Autodesk Inventor part; units mm, degrees
ref_plane "YZ Plane" through (0, 0, 0) normal (1, 0, 0) x (0, 1, 0)
ref_plane "XZ Plane" through (0, 0, 0) normal (0, 1, 0) x (-1, 0, 0)
ref_plane "XY Plane" through (0, 0, 0) normal (0, 0, 1) x (1, 0, 0)
sketch "Sketch1" plane through (0, 0, 0) normal (0, 1, 0) x (-1, 0, 0)
  line L0 (37.5, 25) -> (-37.5, 25)
  line L1 (-37.5, 25) -> (-37.5, -25)
  line L2 (-37.5, -25) -> (37.5, -25)
  line L3 (37.5, -25) -> (37.5, 25)
  circle A0 centre (-7.5, 7.5) radius 1.75
  circle A1 centre (7.5, -7.5) radius 1.75
  line L4 (-7.5, 7.5) -> (7.5, -7.5) construction
  circle A2 centre (15.5, 15.5) radius 5
  line L5 (15.5, 15.5) -> (-15.5, -15.5) construction
  circle A3 centre (-15.5, -15.5) radius 5
  line L6 (15.5, 15.5) -> (13.8367, 7.6748) construction
  line L7 (30.9543, 4.0364) -> (-3.2809, 11.3133) construction
  circle A4 centre (13.8367, 7.6748) radius 14 construction
  line L8 (18.715, -5.4478) -> (4.0428, -2.3291) construction
  line L9 (4.0428, -2.3291) -> (2.9037, -7.6878) construction
  line L10 (2.9037, -7.6878) -> (17.5759, -10.8065) construction
  line L11 (17.5759, -10.8065) -> (18.715, -5.4478) construction
  circle A5 centre (-3.2809, 11.3133) radius 1.75
  circle A6 centre (30.9543, 4.0364) radius 1.75
  line L12 (3.2809, -11.3133) -> (-30.9543, -4.0364) construction
  line L13 (-13.8367, -7.6748) -> (-15.5, -15.5) construction
  circle A7 centre (3.2809, -11.3133) radius 1.75
  circle A8 centre (-30.9543, -4.0364) radius 1.75
  circle A9 centre (-13.8367, -7.6748) radius 14 construction
  line L14 (-4.0428, 2.3291) -> (-18.715, 5.4478) construction
  line L15 (-18.715, 5.4478) -> (-17.5759, 10.8065) construction
  line L16 (-17.5759, 10.8065) -> (-2.9037, 7.6878) construction
  line L17 (-2.9037, 7.6878) -> (-4.0428, 2.3291) construction
  point P0 (0, 0)
  point P1 (0, 0)
  point P2 (0, 25)
  point P3 (-37.5, 0)
  dimension "d0" = 7.5
  dimension "d1" = 7.5
  dimension "d4" = 3.5
  dimension "d6" = 10
  dimension "d7" = 15.5
  dimension "d8" = 15.5
  dimension "d9" = 8
  dimension "d10" = 35
  dimension "d11" = 28
  dimension "d12" = 3.3
  dimension "d13" = 15
  dimension "d14" = 12
  dimension "d15" = 75
  dimension "d16" = 50
extrude "Extrusion1" add sketch "Sketch1" along normal blind 2.5
fillet "Fillet1" radius 25 4 edges at (-37.5, 1.25, 25) (37.5, 1.25, 25) (37.5, 1.25, -25) (-37.5, 1.25, -25)
equation "\"thumbscrew_dia\" = 15.8"
equation "\"helix_length\" = 3.5"
equation "\"helix_width\" = 2"
equation "\"helix_fillet\" = 0.3"
equation "\"helix_inner_dia\" = 19"
equation "\"helix_outer_dia\" = 23"
equation "\"elephant_prevention_radius\" = 0.3"
equation "\"gear_center_distance\" = 25"
equation "\"stepper_screw_dist\" = 35"
equation "\"stepper_axis_offset\" = 8"
equation "\"mount_screw_ortho_dist\" = 31"
equation "\"stepper_dia\" = 28"
equation "\"sheet_thick\" = 2.5"
equation "\"helix_winding_factor\" = 1.2"
properties part number "mount-plate_3DPrint"
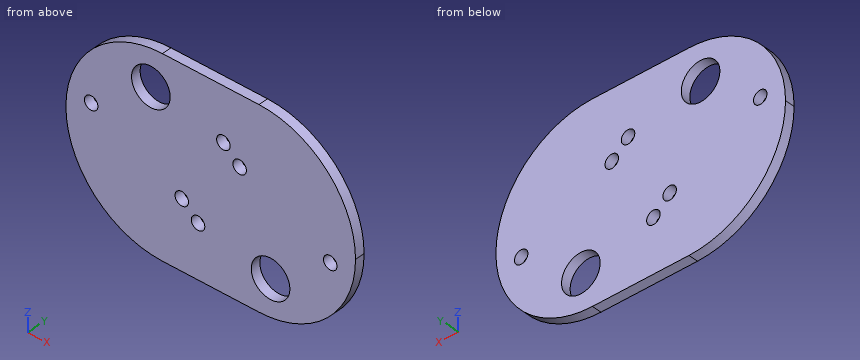
Design review of the part built by this model. Coordinates are the model's own, in mm. Give positions to 0.01 mm unless a question says otherwise; leave off trailing zeros. Order: outer loops, then holes, each group sorted by start corner. A loop starts at its lowest first (then second) coordinate and runs counter-clockwise, first axis right, second up. Notation, with made-up numbers: (-24.75, -26) - (-9.75, -26) arc R6 ccw to (-9.75, -21) - close; hole circle Ø9 at (87, -36.75). An arc over 180 degrees is marked (long way). Use a Markdown table: item, result. Add a question column.
(1) Clearance check with a flat-ended pin moving along its axis: P1, Ø1.5, axis at y = 1, z = -14.5, coming from the -X side. State where the tip first meets the part, or that it passes through.
(2) Add section A-A on x = -7.5. Give the boundary of the cut face in (y, z).
(3) Add section C-C on y = 1. Give the number of separate pieces and of enclosed holes in the cut face, then the cut area to 3 significant figures.
(4) Wall thickness on probe 1 along Z at (x, y) = (7.5, 1.85); probe 2 along Z at (x, y) = (-15.5, 1.45); probe 3 along X at (y, z) = (1.4, -19): over which ranges is each line inside the solid? List them lowest first. Write a range as [from, to].
(5) Add section D-D on x = 23.5. Give the boundary of the cut face in (y, z), then the cut area to 3 significant figures.
(6) Add section B-B on z = 19. Give the boundary of the cut face in (x, y), then the cut area to 3 significant figures.
Report:
| question | item | result |
|---|---|---|
| 1 | P1 | stops at x = -33.38 |
| 2 | outline | (0, -25) - (2.5, -25) - (2.5, -9.25) - (0, -9.25) - close; (0, -5.75) - (2.5, -5.75) - (2.5, 25) - (0, 25) - close |
| 3 | separate pieces | 1 |
| 3 | enclosed holes | 8 |
| 3 | area | 3,000 mm² |
| 4 | probe 1 | z = [-25, 5.75], [9.25, 25] |
| 4 | probe 2 | z = [-24.82, 10.5], [20.5, 24.82] |
| 4 | probe 3 | x = [-28.75, 11.93], [19.07, 28.75] |
| 5 | outline | (0, -22.45) - (2.5, -22.45) - (2.5, 22.45) - (0, 22.45) - close |
| 5 | area | 112 mm² |
| 6 | outline | (-28.75, 0) - (-19.07, 0) - (-19.07, 2.5) - (-28.75, 2.5) - close; (-11.93, 0) - (28.75, 0) - (28.75, 2.5) - (-11.93, 2.5) - close |
| 6 | area | 126 mm² |
